Build history of the part. All positions in model axes, mm. A direction names the side the tool comes from. Coordinates: 2 decimals unless noted, no trailing zeros. Order: outer loops, then holes, each group sorted by start corner. A loop starts at its lowest first (then second) coordinate and runs counter-clockwise, first axis right, second up. Notation, with made-up numbers: (-21, 3) - (6, 3) arc R24 ccw to (6, 22) - close; hole circle Ø3 at (39, 9.25). An arc over 180 degrees is marked (long way). Return JSON: item names as keys, results as strings.
from build123d import *

# Parameters (mm, degrees)
BOSS_EXTRUDE1_DEPTH = 20
CHAMFER1_SIZE       = 5
CHAMFER2_SIZE       = 10
SKETCH2_R           = 1.75
CUT_EXTRUDE1_DEPTH  = 20
SKETCH3_R           = 3
CUT_EXTRUDE2_DEPTH  = 10
BOSS_EXTRUDE2_START = 2
SKETCH4_R           = 3
BOSS_EXTRUDE2_DEPTH = 2
SKETCH5_R           = 1
CUT_EXTRUDE3_DEPTH  = 2
SKETCH6_W           = 12
SKETCH6_H           = 24
CUT_EXTRUDE4_DEPTH  = 12
SKETCH7_W           = 4
SKETCH7_H           = 24
BOSS_EXTRUDE3_DEPTH = 5
CHAMFER3_SIZE       = 5
SKETCH8_W           = 20
SKETCH8_H           = 12
BOSS_EXTRUDE4_DEPTH = 45
SKETCH9_W           = 7
SKETCH9_H           = 20
BOSS_EXTRUDE5_DEPTH = 45
CHAMFER4_SIZE       = 5
CHAMFER5_SIZE       = 7


with BuildPart() as part:
    # Sketch1 → Boss-Extrude1 (new body)
    with BuildSketch(Plane.XY):
        Polygon((16.2, 38.12), (28.2, 38.12), (28.2, -23.88), (-28.8, -23.88), (-28.8, -11.88), (16.2, -11.88), align=None)
    extrude(amount=BOSS_EXTRUDE1_DEPTH)

    # Chamfer1
    chamfer1_edges = [part.edges().sort_by_distance(p)[0] for p in [
        (16.2, -11.88, 10),
    ]]
    chamfer(chamfer1_edges, length=CHAMFER1_SIZE)

    # Chamfer2
    chamfer2_edges = [part.edges().sort_by_distance(p)[0] for p in [
        (28.2, -23.88, 10),
    ]]
    chamfer(chamfer2_edges, length=CHAMFER2_SIZE)

    # Sketch2 → Cut-Extrude1 (cut)
    with BuildSketch(Plane(origin=(0, -11.88, 0), x_dir=(1, 0, 0), z_dir=(0, 1, 0))):
        with Locations(Location((-18.8, -10, 0), (0, 0, 270))):
            Circle(SKETCH2_R)
    extrude(amount=-CUT_EXTRUDE1_DEPTH, mode=Mode.SUBTRACT)

    # Sketch3 → Cut-Extrude2 (cut)
    with BuildSketch(Plane(origin=(0, -11.88, 0), x_dir=(1, 0, 0), z_dir=(0, 1, 0))):
        with Locations(Location((-18.8, -10, 0), (0, 0, 270))):
            Circle(SKETCH3_R)
    extrude(amount=-CUT_EXTRUDE2_DEPTH, mode=Mode.SUBTRACT)

    # Sketch4 → Boss-Extrude2 (add)
    with BuildSketch(Plane(origin=(0, -21.88, 0), x_dir=(1, 0, 0), z_dir=(0, 1, 0)).offset(BOSS_EXTRUDE2_START)):
        with Locations(Location((-18.8, -10, 0), (0, 0, 270))):
            Circle(SKETCH4_R)
    extrude(amount=-BOSS_EXTRUDE2_DEPTH)

    # Sketch5 → Cut-Extrude3 (cut)
    with BuildSketch(Plane(origin=(0, -19.88, 0), x_dir=(1, 0, 0), z_dir=(0, 1, 0))):
        with Locations(Location((-18.8, -10, 0), (0, 0, 270))):
            Circle(SKETCH5_R)
    extrude(amount=-CUT_EXTRUDE3_DEPTH, mode=Mode.SUBTRACT)

    # Sketch6 → Cut-Extrude4 (cut)
    with BuildSketch(Plane.ZY.offset(-16.2)):
        with Locations((10, 16.12)):
            Rectangle(SKETCH6_W, SKETCH6_H)
    extrude(amount=-CUT_EXTRUDE4_DEPTH, mode=Mode.SUBTRACT)

    # Sketch7 → Boss-Extrude3 (add)
    with BuildSketch(Plane(origin=(28.2, 0, 0), x_dir=(0, 0, -1), z_dir=(1, 0, 0))):
        with Locations((-18, 16.12)):
            Rectangle(SKETCH7_W, SKETCH7_H)
        with Locations((-2, 16.12)):
            Rectangle(SKETCH7_W, SKETCH7_H)
    extrude(amount=BOSS_EXTRUDE3_DEPTH)

    # Chamfer3
    chamfer3_edges = [part.edges().sort_by_distance(p)[0] for p in [
        (28.2, 4.12, 18),
        (28.2, 4.12, 2),
        (28.2, 28.12, 18),
        (28.2, 28.12, 2),
    ]]
    chamfer(chamfer3_edges, length=CHAMFER3_SIZE - 0.0001)  # a hair under: the kernel refuses the full size

    # Sketch8 → Boss-Extrude4 (add)
    with BuildSketch(Plane.ZY.offset(28.8)):
        with Locations((10, -17.88)):
            Rectangle(SKETCH8_W, SKETCH8_H)
    extrude(amount=BOSS_EXTRUDE4_DEPTH)

    # Sketch9 → Boss-Extrude5 (add)
    with BuildSketch(Plane(origin=(0, -11.88, 0), x_dir=(1, 0, 0), z_dir=(0, 1, 0))):
        with Locations((-70.3, -10)):
            Rectangle(SKETCH9_W, SKETCH9_H)
    extrude(amount=BOSS_EXTRUDE5_DEPTH)

    # Chamfer4
    chamfer4_edges = [part.edges().sort_by_distance(p)[0] for p in [
        (-66.8, -11.88, 10),
    ]]
    chamfer(chamfer4_edges, length=CHAMFER4_SIZE)

    # Chamfer5
    chamfer5_edges = [part.edges().sort_by_distance(p)[0] for p in [
        (-73.8, -23.88, 10),
    ]]
    chamfer(chamfer5_edges, length=CHAMFER5_SIZE)


solid = part.part
1. Mould opens along Z. For faces 1 (the flat face through (-21, -14, 0)), 2 (the flat face through (30.735, 30.585, 2.028)), 3 (the flat face through (22, 28.12, 10)) say: pulls with the +Z half, pulls with the -Z half, needs draft (parallel to the pull), parting line crosses it, or undercut.
Check values:
{"face 1": "pulls with the -Z half", "face 2": "needs draft", "face 3": "undercut"}
2. Tool access for faces 4 (the flat face through (28.2, -7, 10)), 5 (the flat face through (-18, -19.88, 9)), 6 (the flat face through (13.735, -9.345, 9.86)): list every direction of +Z, -Z, +X, -X, +Y, -Y with a clear straight run to the whole face (end or side of a thin tool).
Check values:
{"face 4": "+X, -Y", "face 5": "+Y", "face 6": "+Z, -Z, +Y"}
3. Cut at A-A on y = 26. Give the cut face in (x, z), plus the area to 3 significant figures.
Check values:
{"outline": "(-73.8, 0) - (-66.8, 0) - (-66.8, 20) - (-73.8, 20) - close; (16.2, 0) - (33.2, 0) - (33.2, 4) - (16.2, 4) - close; (16.2, 16) - (33.2, 16) - (33.2, 20) - (16.2, 20) - close", "area": "276 mm²"}
4. Drop flat-ended pins along their axis: pin 1 (1 mm diameter, centred on x = -52.5, z = 14, fed in from +Y); pin 2 (7.5 mm diameter, centred on x = -71.5, z = 9.5, fed in from +Y). Give the stop position or say it passes through.
Check values:
{"pin 1": "y = -11.88", "pin 2": "y = 33.12"}
5. Cut at C-C on x = -23.5. Give the cut face in (y, z), plus the area to 3 significant figures.
Check values:
{"outline": "(-23.88, 0) - (-11.88, 0) - (-11.88, 20) - (-23.88, 20) - close", "area": "240 mm²"}
6. Probe L1, parallel to X at y = 26.5, z = 16.25; L2, parallel to Z at x = 21, y = 28; L3, parallel to Y at x = 17.5, z = 8.25. List the from-to ranges inside material, lowest first.
Check values:
{"L1": "-73.8 to -66.8, 16.2 to 33.2", "L2": "0 to 4, 16 to 20", "L3": "-23.88 to 4.12, 28.12 to 38.12"}
7. Cut at B-B on z = 5.5. Give the cut face in (x, y).
Check values:
{"outline": "(-73.8, -16.88) - (-66.8, -23.88) - (18.2, -23.88) - (28.2, -13.88) - (28.2, 4.12) - (16.2, 4.12) - (16.2, -6.88) - (11.2, -11.88) - (-61.8, -11.88) - (-66.8, -6.88) - (-66.8, 33.12) - (-73.8, 33.12) - close; (16.2, 28.12) - (28.2, 28.12) - (28.2, 38.12) - (16.2, 38.12) - close"}
